from build123d import *

# Parameters (mm, degrees)
SKETCH1_R           = 5.5
BOSS_EXTRUDE1_DEPTH = 10
SKETCH2_R           = 5
BOSS_EXTRUDE2_DEPTH = 4
SKETCH3_R           = 2.5
BOSS_EXTRUDE3_DEPTH = 8
SKETCH4_R           = 2
BOSS_EXTRUDE4_DEPTH = 10
SKETCH5_R           = 3.75
CUT_EXTRUDE1_DEPTH  = 9
SKETCH6_W           = 25.507413715
SKETCH6_H           = 2.5
CUT_EXTRUDE2_DEPTH  = 10


with BuildPart() as part:
    # Sketch1 → Boss-Extrude1 (new body)
    with BuildSketch(Plane(origin=(0, 0, 0), x_dir=(0, 0, -1), z_dir=(1, 0, 0))):
        Circle(SKETCH1_R)
    extrude(amount=BOSS_EXTRUDE1_DEPTH)

    # Sketch2 → Boss-Extrude2 (add)
    with BuildSketch(Plane(origin=(10, 0, 0), x_dir=(0, 0, -1), z_dir=(1, 0, 0))):
        Circle(SKETCH2_R)
    extrude(amount=BOSS_EXTRUDE2_DEPTH)

    # Sketch3 → Boss-Extrude3 (add)
    with BuildSketch(Plane(origin=(14, 0, 0), x_dir=(0, 0, -1), z_dir=(1, 0, 0))):
        Circle(SKETCH3_R)
    extrude(amount=BOSS_EXTRUDE3_DEPTH)

    # Sketch4 → Boss-Extrude4 (add)
    with BuildSketch(Plane(origin=(22, 0, 0), x_dir=(0, 0, -1), z_dir=(1, 0, 0))):
        Circle(SKETCH4_R)
    extrude(amount=BOSS_EXTRUDE4_DEPTH)

    # Sketch5 → Cut-Extrude1 (cut)
    with BuildSketch(Plane.ZY):
        Circle(SKETCH5_R)
    extrude(amount=-CUT_EXTRUDE1_DEPTH, mode=Mode.SUBTRACT)

    # Sketch6 → Cut-Extrude2 (cut)
    with BuildSketch(Plane.ZY):
        with Locations((1.683379731, 0)):
            Rectangle(SKETCH6_W, SKETCH6_H)
    extrude(amount=-CUT_EXTRUDE2_DEPTH, mode=Mode.SUBTRACT)


solid = part.part
Source: CAD feature listing. Evaluate the final solid. Frame: model axes, mm. A direction names the side the tool comes from. Coordinates: 2 decimals unless noted, no trailing zeros. Loops run counter-clockwise (first coordinate to the right, second up) from the corner with the lowest first, then second, coordinate; pieces in that order, holes last. Notation, with made-up numbers: (62.25, 31.25) - (73.25, 31.25) arc R25 cw to (73.25, 68.25) - close; hole circle Ø5 at (72.5, 74). An arc over 180 degrees is marked (long way). Return JSON: item names as keys, results as strings.
Q1. Mould query, pull axis Y, two halves, no side actions, for faces 6 (the cylindrical face through (4.44, -3.75, -0.06)), 7 (the cylindrical face through (4.9, -5.5, 0.1)), 8 (the flat face through (10, 5.3, 0)). Classes: released by +Y, released by -Y, zero draft, split by the parting line, or undercut.
Results:
{"face 6": "undercut", "face 7": "released by -Y", "face 8": "zero draft"}
Q2. Material intervals for line 1 along X through (y, z) = (4, 1.75); line 2 along Y through (x, z) = (7.5, -3.75); line 3 along Y through (x, z) = (6, 0), sorted ascending.
Results:
{"line 1": "0 to 14", "line 2": "-4.02 to -1.25, 1.25 to 4.02", "line 3": "-5.5 to -3.75, 3.75 to 5.5"}
Q3. Section A-A, the plane x = 4. Return loops of the section in (y, z).
Results:
{"outline": "(-1.25, -5.36) - (-1.25, -3.54) arc R3.75 cw to (-1.25, 3.54) - (-1.25, 5.36) arc R5.5 ccw to start; (1.25, -5.36) arc R5.5 ccw to (1.25, 5.36) - (1.25, 3.54) arc R3.75 cw to (1.25, -3.54) - close"}
Q4. Section B-B, the plane z = 0. Return loops of the section in (x, y), plus the area to 3 significant figures.
Results:
{"outline": "(0, -5.5) - (10, -5.5) - (10, -5) - (14, -5) - (14, -2.5) - (22, -2.5) - (22, -2) - (32, -2) - (32, 2) - (22, 2) - (22, 2.5) - (14, 2.5) - (14, 5) - (10, 5) - (10, 5.5) - (0, 5.5) - (0, 3.75) - (9, 3.75) - (9, 1.25) - (10, 1.25) - (10, -1.25) - (9, -1.25) - (9, -3.75) - (0, -3.75) - close", "area": "160 mm2"}
Q5. Access query for faces 1 (the flat face through (10, -5.3, 0)), 2 (the cylindrical face through (27, -2, 0)), 3 (the flat face through (6, 1.25, -4)), 4 (the flat face through (32, 0, 0)), 5 (the cylindrical face through (4.44, 3.75, 0.06)). Directions: +Z, -Z, +X, -X, +Y, -Y. A direction counts if a zero-diameter tool reaches every point of the face in a straight line with its end or side. Return the directions, or none.
Results:
{"face 1": "+X, -Y", "face 2": "+X", "face 3": "+Z, -Z, -X", "face 4": "+Z, -Z, +X, +Y, -Y", "face 5": "-X"}
Q6. Section D-D, the plane x = 13. Return loops of the section in (y, z), plus the area to 3 significant figures.
Results:
{"outline": "circle Ø10 at (0, 0)", "area": "78.5 mm2"}
Q7. Contact query for flat-ended pins moving along their axis: P1, Ø1.5, axis at x = 24.5, y = -4, coming from the +Z side; P2, Ø2, axis at y = -2.5, z = -1, coming from the -X side; P3, Ø2, axis at y = 4, z = 0.5, coming from the +X side. Output: stop coordinate, or through.
Results:
{"P1": "through", "P2": "x = 9", "P3": "x = 14"}
Q8. Section C-C, the plane y = 0. Return loops of the section in (x, z).
Results:
{"outline": "(10, -5) - (14, -5) - (14, -2.5) - (22, -2.5) - (22, -2) - (32, -2) - (32, 2) - (22, 2) - (22, 2.5) - (14, 2.5) - (14, 5) - (10, 5) - close"}
